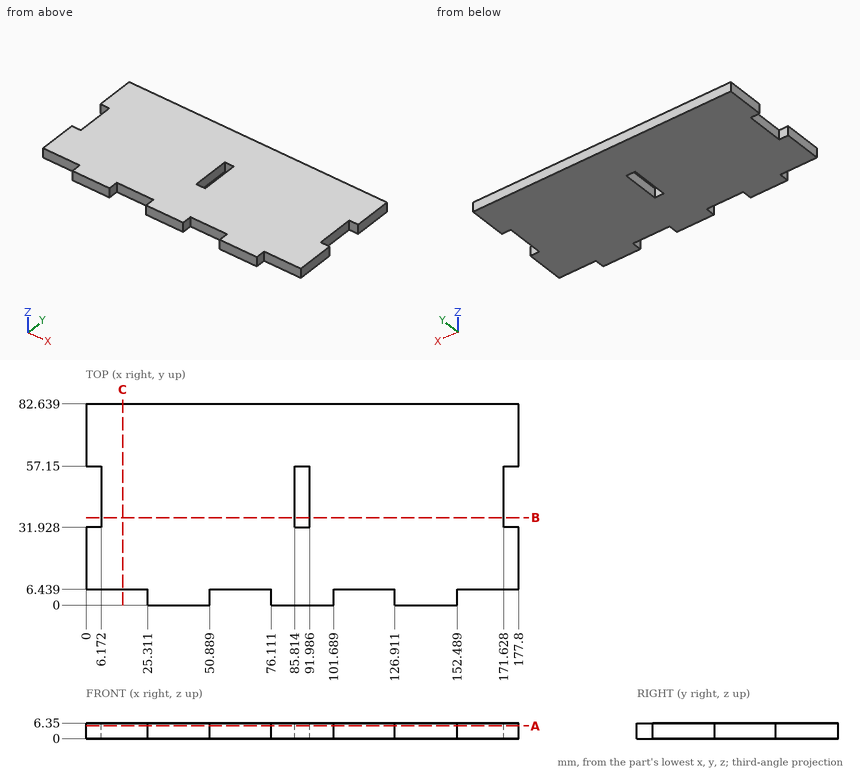
Could you check a few things on this drawing? It's one solid part, dimensions in mm from its lowest x, y, z. Give positions to 0.01 mm unless a question says otherwise; leave off trailing zeros. Loops run counter-clockwise (first coordinate to the right, second up) from the corner with the lowest first, then second, coordinate; pieces in that order, holes last. Notation, with made-up numbers: M -19,4.25 L 16,4.25 A34 cw 16,40.25 Z; hole C 71,29.5 d7. An arc over 180 degrees is marked long. One line per question, with ' | ' between items. Start each with the question number.
Q1. If we section it at C-C (x = 15): Please give me the cut outline in (y, z).
Q2. If we section it at A-A (z = 5.25): Please give me the cut outline in (x, y), plus the area to 3 significant figures.
Q3. For pin 1 Ø1.9 at (x, z) = (114, 2.5) entering from -Y; pin 2 Ø1.5 at (x, y) = (150.5, 40.5) entering from -Z; pin 3 Ø3 at (y, z) = (4, 2.5) entering from -X; pin 4 Ø3 at (y, z) = (50.5, 2) entering from +X, each with a flat end and sliding along its axis, tell me the tip position at first contact or that it passes through.
Q4. If we section it at B-B (y = 36): Please give me the cut outline in (x, z).
Q5. If I drill on line 1 (X direction, y = 57, z = 1.5); line 2 (X direction, y = 5.5, z = 3.25); line 3 (Y direction, x = 15, z = 3.5), over which ranges is the centre line in solid material (lowest first)? Write a range as from..to.
Computed:
1) outline: M 6.44,0 L 82.64,0 L 82.64,6.35 L 6.44,6.35 Z
2) outline: M 0,6.44 L 25.31,6.44 L 25.31,0 L 50.89,0 L 50.89,6.44 L 76.11,6.44 L 76.11,0 L 101.69,0 L 101.69,6.44 L 126.91,6.44 L 126.91,0 L 152.49,0 L 152.49,6.44 L 177.8,6.44 L 177.8,31.93 L 171.63,31.93 L 171.63,57.15 L 177.8,57.15 L 177.8,82.64 L 0,82.64 L 0,57.15 L 6.17,57.15 L 6.17,31.93 L 0,31.93 Z; hole M 85.81,31.93 L 91.99,31.93 L 91.99,57.15 L 85.81,57.15 Z | area: 13,600 mm²
3) pin 1: stops at y = 6.44 | pin 2: stops at z = 0 | pin 3: stops at x = 25.31 | pin 4: stops at x = 171.63
4) outline: M 6.17,0 L 85.81,0 L 85.81,6.35 L 6.17,6.35 Z; M 91.99,0 L 171.63,0 L 171.63,6.35 L 91.99,6.35 Z
5) line 1: x = 6.17..85.81, 91.99..171.63 | line 2: x = 25.31..50.89, 76.11..101.69, 126.91..152.49 | line 3: y = 6.44..82.64
